```python
from build123d import *

# Parameters (mm, degrees)
SKETCH1_R           = 2.1
BOSS_EXTRUDE1_DEPTH = 5
SKETCH2_R           = 1.4
CUT_EXTRUDE1_DEPTH  = 145.546048026


with BuildPart() as part:
    # Sketch1 → Boss-Extrude1 (new body)
    with BuildSketch(Plane.XY):
        with BuildLine():
            Line((41, 136.6), (41, 125.6))
            ThreePointArc((41, 125.6), (41.878679656, 123.478679656), (44, 122.6))
            Line((44, 122.6), (47, 122.6))
            Line((47, 122.6), (47, -29.8))
            Line((47, -29.8), (47, -58.8))
            Line((47, -58.8), (43.5, -58.8))
            Line((43.5, -58.8), (43.5, -63.8))
            Line((43.5, -63.8), (10, -63.8))
            Line((10, -63.8), (10, -58.8))
            Line((10, -58.8), (-12.5, -58.8))
            Line((-12.5, -58.8), (-12.5, 0))
            ThreePointArc((-12.5, 0), (-8.838834765, 8.838834765), (0, 12.5))
            Line((0, 12.5), (16, 12.5))
            Line((16, 12.5), (16, 104.5))
            Line((16, 104.5), (0, 104.5))
            ThreePointArc((0, 104.5), (-8.838834765, 108.161165235), (-12.5, 117))
            Line((-12.5, 117), (-12.5, 124.1))
            ThreePointArc((-12.5, 124.1), (-8.838834765, 132.938834765), (0, 136.6))
            Line((0, 136.6), (37.5, 136.6))
            Line((37.5, 136.6), (41, 136.6))
        make_face()
        Circle(SKETCH1_R, mode=Mode.SUBTRACT)
        with Locations((0, 117)):
            Circle(SKETCH1_R, mode=Mode.SUBTRACT)
    extrude(amount=BOSS_EXTRUDE1_DEPTH)

    # Sketch2 → Cut-Extrude1 (cut, through all)
    with BuildSketch(Plane.XY.offset(5)):
        with Locations((13.2, -21.3)):
            Circle(SKETCH2_R)
        with Locations((24.5, 134)):
            Circle(SKETCH2_R)
    extrude(amount=-CUT_EXTRUDE1_DEPTH, mode=Mode.SUBTRACT)


solid = part.part
```
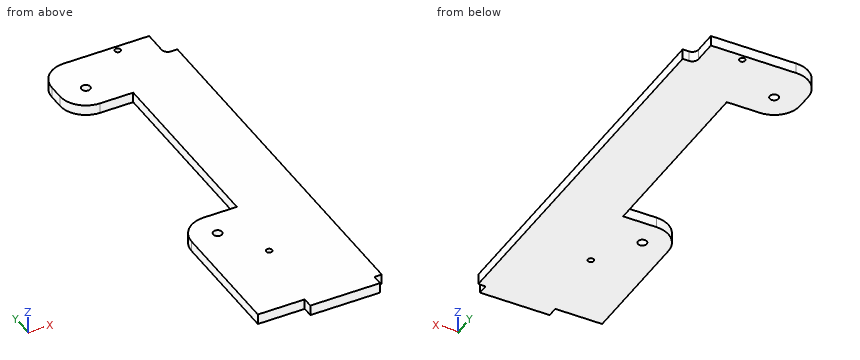
Work out the finished part from the listing and answer in its coordinate system (mm). Give positions to 0.01 mm unless a question says otherwise; leave off trailing zeros. Order: outer loops, then holes, each group sorted by start corner. A loop starts at its lowest first (then second) coordinate and runs counter-clockwise, first axis right, second up. Notation, with made-up numbers: M -9,-35.5 L 31,-35.5 A14 cw 31,-8.5 Z; hole C 26,47.5 d10. An arc over 180 degrees is marked long. Return JSON: item names as keys, results as strings.
1) Each of these flat-tipped pins is pushed along its axis until it touches: pin 1 (2.5 mm diameter, centred on x = 5, z = 1.5, fed in from -Y); pin 2 (2.5 mm diameter, centred on x = 0, y = 0, fed in from -Z); pin 3 (1.5 mm diameter, centred on y = -60.5, z = 3, fed in from +X); pin 4 (2.5 mm diameter, centred on y = 132.5, z = 2, fed in from +X). Where does it stop, or does it pass through?
Resolved:
{"pin 1": "y = -58.8", "pin 2": "through", "pin 3": "x = 43.5", "pin 4": "x = 41"}
2) Section B-B, the plane y = 31.5 is taken. Write down the section's boundary in (x, z).
Resolved:
{"outline": "M 16,0 L 47,0 L 47,5 L 16,5 Z"}
3) Straight lines are drawn through the part: line 1 along Y through (x, z) = (0, 2.2); line 2 along Y through (x, z) = (13.2, 3.75); line 3 along Y through (x, z) = (6, 3.55). For each, find the intervals that lie inside material, in ascending order. Write a range as [from, to].
Resolved:
{"line 1": "[-58.8, -2.1], [2.1, 12.5], [104.5, 114.9], [119.1, 136.6]", "line 2": "[-63.8, -22.7], [-19.9, 12.5], [104.5, 136.6]", "line 3": "[-58.8, 12.5], [104.5, 136.6]"}
4) Section C-C, the plane y = 9 is taken. Write down the section's boundary in (x, z), plus the area to 3 significant figures.
Resolved:
{"outline": "M -8.67,0 L 47,0 L 47,5 L -8.67,5 Z", "area": "278 mm^2"}
5) Section A-A, the plane z = 2.4 is taken. Write down the section's boundary in (x, y), plus the area to 3 significant figures.
Resolved:
{"outline": "M -12.5,-58.8 L 10,-58.8 L 10,-63.8 L 43.5,-63.8 L 43.5,-58.8 L 47,-58.8 L 47,122.6 L 44,122.6 A3 cw 41,125.6 L 41,136.6 L 0,136.6 A12.5 ccw -12.5,124.1 L -12.5,117 A12.5 ccw 0,104.5 L 16,104.5 L 16,12.5 L 0,12.5 A12.5 ccw -12.5,0 Z; hole C 0,0 d4.2; hole C 0,117 d4.2; hole C 13.2,-21.3 d2.8; hole C 24.5,134 d2.8", "area": "8,950 mm^2"}
